Verification items for the finished model (mm, model axes). Face numbers are marked on the shaded views. A direction names the side the tool comes from. Round coordinates to 2 decimals unless told otherwise and drop trailing zeros. Order: outer loops, then holes, each group sorted by start corner. A loop starts at its lowest first (then second) coordinate and runs counter-clockwise, first axis right, second up. Notation, with made-up numbers: M 59,-3.5 L 99,-3.5 A17 ccw 99,0.5 Z; hole C 62.5,64 d4. An arc over 180 degrees is marked long. Use one line per item in the form item = value. Start each with the question number.
Item 1: Go/stop test with flat-tipped pins: pin 1 Ø4 at (x, z) = (-2.5, 6) entering from +Y; pin 2 Ø5.5 at (y, z) = (11, 7.5) entering from +X (3 decimals); pin 3 Ø8 at (x, y) = (-11, 10) entering from -Z; pin 4 Ø4 at (y, z) = (13.5, 6.5) entering from +X. Record where each tip stops, or that it passes through.
Item 2: Thickness scan on probe 1 along Y at (x, z) = (0, 4.25) (1 decimal); probe 2 along Y at (x, z) = (-8.25, 4.25) (1 decimal); probe 3 along X at (y, z) = (17.5, 4.5) (3 decimals). Record the ranges inside material, lowest first. Write a range as [from, to].
Item 3: Release check for a two-part mould opening along Y. For the marked faces 1, 2, 3 and 4 record: +Y half, -Y half, draft (parallel to the pull), parting line (faces both ways), or undercut.
Item 4: Cross-section at A-A on z = 6.35. Count the separate pieces of the cut face and the enclosed holes in it, then the cut area to 3 significant figures.
Item 5: Cross-section at B-B on x = 0. Enter the section's corners in (y, z) (1 decimal).
Item 6: Tool access check on the marked faces 5, 6 and 7. Record the directions out of +Z, -Z, +X, -X, +Y, -Y that give a thin tool (end or side, any length) a straight path to the whole face; none if there is none.
from build123d import *

# Parameters (mm, degrees)
F0_R      = 4.7625
F1_DEPTH  = 12.7
F2_R      = 6.35
F3_R      = 3.175
F4_R      = 1.8415
F5_DEPTH  = 25.4
F7_DEPTH  = 3.175
F8_R      = 1.8415
F9_DEPTH  = 25.4
F11_DEPTH = 3.175
F12_W     = 20.617577
F12_H     = 29.730969
F13_DEPTH = 25.4
F14_R     = 3.175


with BuildPart() as f1:
    # F0 (on Top) → F1 (new body)
    with BuildSketch(Plane.XY):
        Polygon((-13.335, 18.415), (-13.335, -13.335), (18.415, -13.335), (18.415, -6.985), (7.62, -6.985), (7.62, 7.62), (-6.985, 7.62), (-6.985, 18.415), align=None)
        Circle(F0_R, mode=Mode.SUBTRACT)
    extrude(amount=F1_DEPTH)

    # F2
    f2_edges = [f1.edges().sort_by_distance(p)[0] for p in [
        (7.62, 7.62, 6.35),
    ]]
    fillet(f2_edges, radius=F2_R)

    # F3
    f3_edges = [f1.edges().sort_by_distance(p)[0] for p in [
        (-13.335, -13.335, 6.35),
    ]]
    fillet(f3_edges, radius=F3_R)

    # F4 (on face) → F5 (cut)
    with BuildSketch(Plane(origin=(0, -6.985, 0), x_dir=(-1, 0, 0), z_dir=(0, 1, 0))):
        with Locations((-13.0175, 6.35)):
            Circle(F4_R)
    extrude(amount=-F5_DEPTH, mode=Mode.SUBTRACT)

    # F6 (on face) → F7 (cut)
    with BuildSketch(Plane(origin=(0, -6.985, 0), x_dir=(-1, 0, 0), z_dir=(0, 1, 0))):
        Polygon((-17.0815, 4.003649), (-13.0175, 1.657297), (-8.9535, 4.003649), (-8.9535, 8.696351), (-13.0175, 11.042703), (-17.0815, 8.696351), align=None)
    extrude(amount=-F7_DEPTH, mode=Mode.SUBTRACT)

    # F8 (on face) → F9 (cut)
    with BuildSketch(Plane.YZ.offset(-6.985)):
        with Locations((13.0175, 6.35)):
            Circle(F8_R)
    extrude(amount=-F9_DEPTH, mode=Mode.SUBTRACT)

    # F10 (on face) → F11 (cut)
    with BuildSketch(Plane.YZ.offset(-6.985)):
        Polygon((8.9535, 8.696351), (8.9535, 4.003649), (13.0175, 1.657297), (17.0815, 4.003649), (17.0815, 8.696351), (13.0175, 11.042703), align=None)
    extrude(amount=-F11_DEPTH, mode=Mode.SUBTRACT)

    # F12 (on face) → F13 (cut)
    with BuildSketch(Plane.XY.offset(12.7)):
        with Locations((17.928788, -6.337149)):
            Rectangle(F12_W, F12_H)
    extrude(amount=-F13_DEPTH, mode=Mode.SUBTRACT)

    # F14
    f14_edges = [f1.edges().sort_by_distance(p)[0] for p in [
        (7.62, -13.335, 6.35),
    ]]
    fillet(f14_edges, radius=F14_R)


solid = f1.part
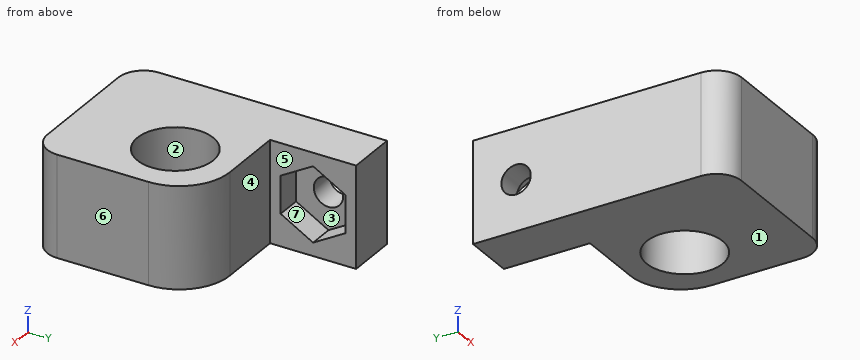
Output values:
q1.pin_1 = 7.62
q1.pin_2 = -6.985
q1.pin_3 = 0
q1.pin_4 = -10.16
q2.probe_1 = [-13.3, -4.8], [4.8, 7.6]
q2.probe_2 = [-13.3, 9], [17.1, 18.4]
q2.probe_3 = [-13.335, -6.985]
q3.face_1 = draft
q3.face_2 = undercut
q3.face_3 = undercut
q3.face_4 = +Y half
q4.separate_pieces = 2
q4.enclosed_holes = 1
q4.area = 386 mm2
q5.outline = M -13.3,0 L -4.8,0 L -4.8,12.7 L -13.3,12.7 Z; M 4.8,0 L 7.6,0 L 7.6,12.7 L 4.8,12.7 Z
q6.face_5 = +Z, -Z, +X, +Y
q6.face_6 = +Z, -Z, +X, +Y, -Y
q6.face_7 = +X
